```python
from build123d import *

# Parameters (mm, degrees)
EXTRUDE_1_DEPTH = 3
EXTRUDE_2_DEPTH = 8


with BuildPart() as part:
    # Sketch 1 → Extrude 1 (new body)
    # profile 1 of 2: a face of its own
    with BuildSketch(Plane(origin=(0, 0, 0), x_dir=(1, 0, 0), z_dir=(0, 1, 0))):
        with BuildLine():
            Line((0, 25), (0, -80))
            ThreePointArc((0, -80), (56.568542495, -56.568542495), (80, 0))
            ThreePointArc((80, 0), (56.568542495, 56.568542495), (0, 80))
            Line((0, 80), (0, 26.5))
            ThreePointArc((0, 26.5), (22.066574498, 38.749862186), (23.339880034, 63.956439237))
            Line((23.339880034, 63.956439237), (25, 63.956439237))
            ThreePointArc((25, 63.956439237), (23.14413618, 37.647425796), (0, 25))
        make_face()
        with BuildLine():
            ThreePointArc((56.475011367, -38.023008969), (15.576309186, -21.438950351), (18.710292179, -65.460683517))
            Line((18.710292179, -65.460683517), (17.367226914, -66.43647755))
            ThreePointArc((17.367226914, -66.43647755), (14.694631307, -20.225424859), (57.818076632, -37.047214935))
            Line((57.818076632, -37.047214935), (56.475011367, -38.023008969))
        make_face(mode=Mode.SUBTRACT)
        with BuildLine():
            ThreePointArc((53.613768719, 41.96117162), (25.202997682, 8.188950351), (68.038607873, -2.433918372))
            Line((68.038607873, -2.433918372), (68.551613155, -4.012786283))
            ThreePointArc((68.551613155, -4.012786283), (23.776412907, 7.725424859), (53.100763436, 43.540039531))
            Line((53.100763436, 43.540039531), (53.613768719, 41.96117162))
        make_face(mode=Mode.SUBTRACT)
    # profile 2 of 2: a face of its own
    with BuildSketch(Plane(origin=(0, 0, 0), x_dir=(1, 0, 0), z_dir=(0, 1, 0))):
        with BuildLine():
            ThreePointArc((0, 80), (-80, 0), (0, -80))
            Line((0, -80), (0, 25))
            ThreePointArc((0, 25), (-23.14413618, 37.647425796), (-25, 63.956439237))
            Line((-25, 63.956439237), (-23.339880034, 63.956439237))
            ThreePointArc((-23.339880034, 63.956439237), (-22.066574498, 38.749862186), (0, 26.5))
            Line((0, 26.5), (0, 80))
        make_face()
        with BuildLine():
            ThreePointArc((-18.710292179, -65.460683517), (-15.576309186, -21.438950351), (-56.475011367, -38.023008969))
            Line((-56.475011367, -38.023008969), (-57.818076632, -37.047214935))
            ThreePointArc((-57.818076632, -37.047214935), (-14.694631307, -20.225424859), (-17.367226914, -66.43647755))
            Line((-17.367226914, -66.43647755), (-18.710292179, -65.460683517))
        make_face(mode=Mode.SUBTRACT)
        with BuildLine():
            ThreePointArc((-68.038607873, -2.433918372), (-25.202997682, 8.188950351), (-53.613768719, 41.96117162))
            Line((-53.613768719, 41.96117162), (-53.100763436, 43.540039531))
            ThreePointArc((-53.100763436, 43.540039531), (-23.776412907, 7.725424859), (-68.551613155, -4.012786283))
            Line((-68.551613155, -4.012786283), (-68.038607873, -2.433918372))
        make_face(mode=Mode.SUBTRACT)
    extrude(amount=EXTRUDE_1_DEPTH)

    # Sketch 1_5 → Extrude 2 (add)
    with BuildSketch(Plane(origin=(0, 0, 0), x_dir=(1, 0, 0), z_dir=(0, 1, 0))):
        with BuildLine():
            Line((-25, 63.956439237), (-23.339880034, 63.956439237))
            ThreePointArc((-23.339880034, 63.956439237), (0, 26.5), (23.339880034, 63.956439237))
            Line((23.339880034, 63.956439237), (25, 63.956439237))
            ThreePointArc((25, 63.956439237), (0, 25), (-25, 63.956439237))
        make_face()
        with BuildLine():
            Line((68.038607873, -2.433918372), (68.551613155, -4.012786283))
            ThreePointArc((68.551613155, -4.012786283), (23.776412907, 7.725424859), (53.100763436, 43.540039531))
            Line((53.100763436, 43.540039531), (53.613768719, 41.96117162))
            ThreePointArc((53.613768719, 41.96117162), (25.202997682, 8.188950351), (68.038607873, -2.433918372))
        make_face()
        with BuildLine():
            Line((18.710292179, -65.460683517), (17.367226914, -66.43647755))
            ThreePointArc((17.367226914, -66.43647755), (14.694631307, -20.225424859), (57.818076632, -37.047214935))
            Line((57.818076632, -37.047214935), (56.475011367, -38.023008969))
            ThreePointArc((56.475011367, -38.023008969), (15.576309186, -21.438950351), (18.710292179, -65.460683517))
        make_face()
        with BuildLine():
            Line((-56.475011367, -38.023008969), (-57.818076632, -37.047214935))
            ThreePointArc((-57.818076632, -37.047214935), (-14.694631307, -20.225424859), (-17.367226914, -66.43647755))
            Line((-17.367226914, -66.43647755), (-18.710292179, -65.460683517))
            ThreePointArc((-18.710292179, -65.460683517), (-15.576309186, -21.438950351), (-56.475011367, -38.023008969))
        make_face()
        with BuildLine():
            Line((-53.613768719, 41.96117162), (-53.100763436, 43.540039531))
            ThreePointArc((-53.100763436, 43.540039531), (-23.776412907, 7.725424859), (-68.551613155, -4.012786283))
            Line((-68.551613155, -4.012786283), (-68.038607873, -2.433918372))
            ThreePointArc((-68.038607873, -2.433918372), (-25.202997682, 8.188950351), (-53.613768719, 41.96117162))
        make_face()
    extrude(amount=EXTRUDE_2_DEPTH)


solid = part.part
```
Can you work these out from the model? Positions are in its coordinate system, mm. A direction names the side the tool comes from. Give positions to 0.01 mm unless a question says otherwise; leave off trailing zeros. Write each loop counter-clockwise with the first axis right and the second up, starting at its lowest first coordinate (ties: lowest second). Pieces come first, ordered by that corner, then holes. Notation, with made-up numbers: (54, -14) -> (94, -14) arc R20 cw to (94, 18) -> close; hole circle Ø9 at (18, 52). An arc over 180 degrees is marked (long way). Write item = value, one per line.
(1) Suppose I cut it at D-D on x = -65.5. Write out the boundary of the cut face in (y, z), then the cut area to 3 significant figures.
Worked out:
outline = (0, -45.93) -> (3, -45.93) -> (3, 4.6) -> (8, 4.6) -> (8, 6.44) -> (3, 6.44) -> (3, 45.93) -> (0, 45.93) -> close
area = 285 mm^2
(2) I'm going to push flat-ended pins straight in: P1, Ø1, axis at y = 2, z = 1.5, coming from the -X side; P2, Ø12, axis at x = -28, z = 1.5, coming from the +Y side; P3, Ø1.8, axis at x = 24, y = 5.5, coming from the -Z side; P4, Ø4, axis at y = 3, z = 51.5, coming from the -X side. Where does each tip first touch, or does it pass through?
Worked out:
P1 = -79.99
P2 = 8
P3 = -63.96
P4 = -62.85
(3) Suppose I cut it at B-B on x = 51. Write out the boundary of the cut face in (y, z).
Worked out:
outline = (0, -61.64) -> (3, -61.64) -> (3, -43.7) -> (8, -43.7) -> (8, -42.2) -> (3, -42.2) -> (3, 9.75) -> (8, 9.75) -> (8, 11.26) -> (3, 11.26) -> (3, 23.75) -> (8, 23.75) -> (8, 26.03) -> (3, 26.03) -> (3, 61.64) -> (0, 61.64) -> close
(4) For faces 4 (the face through (-14, 8, 22)), 5 (the face through (0.77, 5.46, -25.01)), which set-ups out of +Z, -Z, +X, -X, +Y, -Y let a thin tool reach every point of the face, with its end or its side?
Worked out:
face_4 = +Z, -Z, +X, -X, +Y
face_5 = +Y
(5) Suppose I cut it at A-A on y = 6. Write out the boundary of the cut face in (x, z), then the cut area to 3 significant figures.
Worked out:
outline = (-68.55, 4.01) -> (-68.04, 2.43) arc R26 cw (long way) to (-53.61, -41.96) -> (-53.1, -43.54) arc R27.5 ccw (long way) to start; (-57.82, 37.05) arc R27.5 ccw (long way) to (-17.37, 66.44) -> (-18.71, 65.46) arc R26 cw (long way) to (-56.48, 38.02) -> close; (-25, -63.96) -> (-23.34, -63.96) arc R26 cw (long way) to (23.34, -63.96) -> (25, -63.96) arc R27.5 ccw (long way) to start; (17.37, 66.44) arc R27.5 ccw (long way) to (57.82, 37.05) -> (56.48, 38.02) arc R26 cw (long way) to (18.71, 65.46) -> close; (53.1, -43.54) -> (53.61, -41.96) arc R26 cw (long way) to (68.04, 2.43) -> (68.55, 4.01) arc R27.5 ccw (long way) to start
area = 808 mm^2
(6) I need wall thicknesses on probe 1 along Z at (x, y) = (10, 3.75); probe 2 along Z at (x, y) = (35, 5.25); probe 3 along X at (y, z) = (7, 30). Which ranges of each line are inside material? Lowest first, please. Write a range as from..to.
Worked out:
probe_1 = -28.5..-26.88, 24.55..26.95, 57.99..60.39
probe_2 = -39.32..-37.51, 5.06..6.87, 15.29..16.81
probe_3 = -55.37..-53.67, -8.05..-6.35, 6.35..8.05, 53.67..55.37
(7) Thinking about a two-plate mould opening in Z: for faces 1 (the face through (-14.99, 5.46, 21.88)), 2 (the face through (-23.55, 5.46, -8.46)), 3 (the face through (-25, 8, -8)), which applies, released by +Z, released by -Z, zero draft, split by the parting line, or undercut?
Worked out:
face_1 = undercut
face_2 = undercut
face_3 = zero draft
(8) Suppose I cut it at C-C on z = -52.5. Write out the boundary of the cut face in (x, y), then the cut area to 3 significant figures.
Worked out:
outline = (-60.36, 0) -> (60.36, 0) -> (60.36, 3) -> (27.5, 3) -> (27.5, 8) -> (26, 8) -> (26, 3) -> (-26, 3) -> (-26, 8) -> (-27.5, 8) -> (-27.5, 3) -> (-60.36, 3) -> close
area = 377 mm^2
